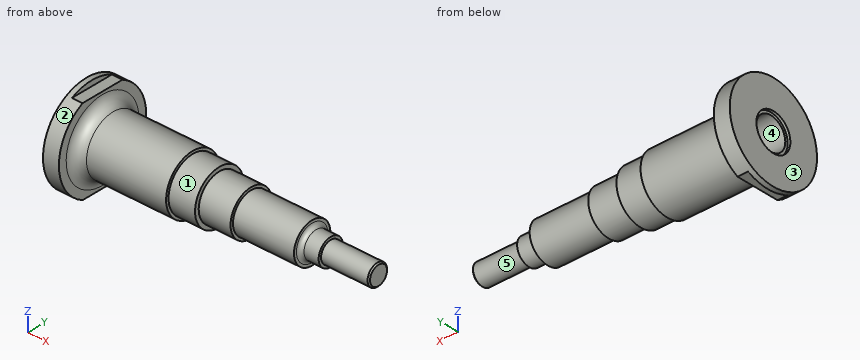
```python
from build123d import *

# Parameters (mm, degrees)
ESQUISSE3_W             = 4
ESQUISSE3_H             = 20
ENL_V_MAT_EXTRU_1_DEPTH = 4


with BuildPart() as part:
    # Esquisse1 → Base-Révolution (revolve)
    with BuildSketch(Plane.XY, mode=Mode.PRIVATE) as base_r_volution_sk:
        with BuildLine():
            Line((-130, 7), (-130, 18))
            Line((-130, 18), (-124, 18))
            Line((-124, 18), (-124, 15))
            ThreePointArc((-124, 15), (-122.828427125, 12.171572875), (-120, 11))
            Line((-120, 11), (-90, 11))
            Line((-90, 11), (-90, 10))
            Line((-90, 10), (-80, 10))
            Line((-80, 10), (-80, 8.5))
            Line((-80, 8.5), (-68, 8.5))
            Line((-68, 8.5), (-68, 7.5))
            Line((-68, 7.5), (-45, 7.5))
            Line((-45, 7.5), (-45, 6.5))
            ThreePointArc((-45, 6.5), (-44.560660172, 5.439339828), (-43.5, 5))
            Line((-43.5, 5), (-38, 5))
            Line((-38, 5), (-38, 4))
            Line((-38, 4), (-20.461275116, 4))
            Line((-20.461275116, 4), (-20, 3.5))
            Line((-20, 3.5), (-20, 0))
            Line((-20, 0), (-92.003246889, 0))
            Line((-92.003246889, 0), (-95.003246889, 5))
            Line((-95.003246889, 5), (-101.003246889, 5))
            Line((-101.003246889, 5), (-101.003246889, 6))
            Line((-101.003246889, 6), (-129.003246889, 6))
            Line((-129.003246889, 6), (-129.003246889, 7))
            Line((-129.003246889, 7), (-130, 7))
        make_face()
    revolve(base_r_volution_sk.sketch.rotate(Axis((-125, 0, 0), (1, 0, 0)), 90), axis=Axis((-125, 0, 0), (1, 0, 0)))

    # Esquisse3 → Enlèv. mat.-Extru.1 (cut)
    with BuildSketch(Plane(origin=(-124, 0, 0), x_dir=(0, 0, -1), z_dir=(1, 0, 0))):
        with Locations((-18, 0)):
            Rectangle(ESQUISSE3_W, ESQUISSE3_H)
        with Locations((18, 0)):
            Rectangle(ESQUISSE3_W, ESQUISSE3_H)
    extrude(amount=-ENL_V_MAT_EXTRU_1_DEPTH, mode=Mode.SUBTRACT)


solid = part.part
```
Can you work these out from the model? Positions are in its coordinate system, mm. Face numbers are marked on the shaded views. A direction names the side the tool comes from. Give positions to 0.01 mm unless a question says otherwise; leave off trailing zeros. Loops run counter-clockwise (first coordinate to the right, second up) from the corner with the lowest first, then second, coordinate; pieces in that order, holes last. Notation, with made-up numbers: M 73.5,24 L 130.5,24 A18 cw 130.5,40 Z; hole C -29.75,64.5 d8. An arc over 180 degrees is marked long. One line per question, with ' | ' between items. Start each with the question number.
Q1. For the marked faces 1 and 2, which set-ups out of +Z, -Z, +X, -X, +Y, -Y let a thin tool reach every point of the face, with its end or its side?
Q2. If we section it at B-B (x = -59): Please give me the cut outline in (y, z), plus the area to 3 significant figures.
Q3. If we mould it in two halves opening along Y, with no side actions, what happens to the marked faces 3, 4 and 5? For each: +Y half, -Y half, draft (parallel to the pull), parting line (faces both ways), or undercut.
Q4. If we section it at A-A (x = -104.5): Please give me the cut outline in (y, z), plus the area to 3 significant figures.
Q5. If I drill on line 1 (Y direction, x = -99.8, z = 0); line 2 (X direction, y = 4.5, z = -7); line 3 (X direction, y = 13, z = 7), over which ranges is the centre line in solid material (lowest first)? Write a range as from..to.
Q6. For pin 1 Ø1.5 at (x, y) = (-94, -9) entering from -Z; pin 2 Ø9.5 at (y, z) = (-8, 1) entering from +X; pin 3 Ø11 at (y, z) = (0, 0) entering from -X; pin 4 Ø1 at (y, z) = (-3, -17) entering from +X, each with a flat end and sliding along its axis, tell me the tip position at first contact or that it passes through.
Q7. If we section it at C-C (x = -42.5): Please give me the cut outline in (y, z), plus the area to 3 significant figures.
Computed:
1) face 1: +X | face 2: +X, -X
2) outline: C 0,0 d15 | area: 177 mm²
3) face 3: draft | face 4: undercut | face 5: parting line
4) outline: C 0,0 d22; hole C 0,0 d12 | area: 267 mm²
5) line 1: y = -11..-5, 5..11 | line 2: x = -130..-68 | line 3: x = -130..-123.99
6) pin 1: stops at z = -7.28 | pin 2: stops at x = -20 | pin 3: stops at x = -101 | pin 4: stops at x = -128
7) outline: C 0,0 d10 | area: 78.5 mm²
